```python
from build123d import *

# Parameters (mm, degrees)
F0_R      = 40
F1_DEPTH  = 20
F2_R      = 25
F3_DEPTH  = 40
F4_R      = 20
F5_DEPTH  = 40
F6_R      = 25
F7_DEPTH  = 20
F8_R      = 20
F9_DEPTH  = 20
F11_R     = 10
F12_DEPTH = 20
F13_R     = 5
F14_DEPTH = 20
F15_R     = 2.5
F16_DEPTH = 20


with BuildPart() as f1:
    # F0 (on Front) → F1 (new body)
    with BuildSketch(Plane.XZ):
        Circle(F0_R)
    extrude(amount=F1_DEPTH)

    # F2 (on face) → F3 (join)
    with BuildSketch(Plane.XZ.offset(20)):
        Circle(F2_R)
    extrude(amount=F3_DEPTH)

    # F4 (on face) → F5 (cut)
    with BuildSketch(Plane.XZ.offset(60)):
        Circle(F4_R)
    extrude(amount=-F5_DEPTH, mode=Mode.SUBTRACT)

    # F6 (on face) → F7 (join)
    with BuildSketch(Plane(origin=(0, 0, 0), x_dir=(-1, 0, 0), z_dir=(0, 1, 0))):
        Circle(F6_R)
    extrude(amount=F7_DEPTH)

    # F8 (on face) → F9 (join)
    with BuildSketch(Plane(origin=(0, 20, 0), x_dir=(-1, 0, 0), z_dir=(0, 1, 0))):
        Circle(F8_R)
    extrude(amount=F9_DEPTH)

    # F11 (on face) → F12 (join)
    with BuildSketch(Plane(origin=(0, 40, 0), x_dir=(-1, 0, 0), z_dir=(0, 1, 0))):
        Circle(F11_R)
    extrude(amount=F12_DEPTH)

    # F13 (on face) → F14 (join)
    with BuildSketch(Plane(origin=(0, 60, 0), x_dir=(-1, 0, 0), z_dir=(0, 1, 0))):
        Circle(F13_R)
    extrude(amount=F14_DEPTH)

    # F15 (on face) → F16 (join)
    with BuildSketch(Plane(origin=(0, 80, 0), x_dir=(-1, 0, 0), z_dir=(0, 1, 0))):
        Circle(F15_R)
    extrude(amount=F16_DEPTH)


solid = f1.part
```
Design review of the part built by this model. Coordinates are the model's own, in mm. A direction names the side the tool comes from. Coordinates: 2 decimals unless noted, no trailing zeros. Order: outer loops, then holes, each group sorted by start corner. A loop starts at its lowest first (then second) coordinate and runs counter-clockwise, first axis right, second up. Notation, with made-up numbers: (46, 68.5) -> (100, 68.5) arc R20 cw to (100, 101.5) -> close; hole circle Ø1 at (47.25, -26). An arc over 180 degrees is marked (long way). One line per item, written item: value. Start each with the question number.
Q1. Tool access review of faces 4 (the cylindrical face through (-4.336, -40.28, -19.524)), 5 (the flat face through (-11, -60, 17)), 6 (the cylindrical face through (0.54, 89.86, -2.44)): name each direction out of +Z, -Z, +X, -X, +Y, -Y from which nothing blocks a thin tool from reaching the whole face with its end or side.
Q2. Take a section at C-C, the plane y = -33. State the section outline as (x, z) points.
Q3. Insertion check: pin 1 Ø3 at (y, z) = (3, -22.5) entering from -X; pin 2 Ø1.5 at (y, z) = (-15.5, 28) entering from +X; pin 3 Ø10 at (y, z) = (-43, 22) entering from -X; pin 4 Ø6 at (x, z) = (-3, 3) entering from +Y. Each pin has a flat end and moves straight along its axis. Give the tip position at first contact, or say it passes through.
Q4. Take a section at D-D, the plane y = 7. State the section outline as (x, z) points.
Q5. Mouldability with a two-part tool opening along Z and no side actions: class faces 1 (the flat face through (0, -20, 0)), 2 (the flat face through (17.22, 0, 18.34)), 3 (the cylindrical face through (2.17, 49.86, -9.76)) as pulls with the +Z half, pulls with the -Z half, needs draft (parallel to the pull), parting line crosses it, or undercut.
Q6. For probe 1 along Z at (x, y) = (0, -28); probe 2 along Y at (x, z) = (23, 11); probe 3 along Z at (x, y) = (-0.5, 13.5) (3 decimals), list the stretches that pass through material, from the lowest coordinate up.
Values follow:
1. face 4: -Y
1. face 5: +Z, -Z, +X, -X, -Y
1. face 6: +Y
2. outline: circle Ø50 at (0, 0); hole circle Ø40 at (0, 0)
3. pin 1: stops at x = -13.56
3. pin 2: stops at x = 29.28
3. pin 3: stops at x = -18.33
3. pin 4: stops at y = 100
4. outline: circle Ø50 at (0, 0)
5. face 1: undercut
5. face 2: needs draft
5. face 3: parting line crosses it
6. probe 1: z = -25 to -20, 20 to 25
6. probe 2: y = -20 to 0
6. probe 3: z = -24.995 to 24.995
